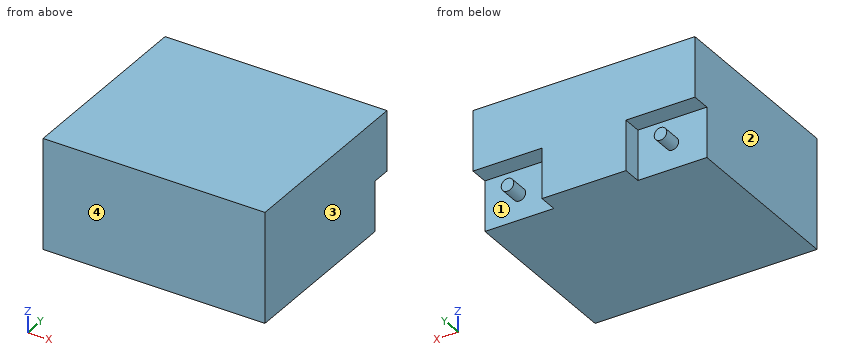
from build123d import *

# Parameters (mm, degrees)
F0_W     = 177
F0_H     = 154
F1_DEPTH = 88
F2_W     = 55
F2_H     = 40
F2_R     = 5
F3_DEPTH = 15


with BuildPart() as f1:
    # F0 (on Top) → F1 (new body)
    with BuildSketch(Plane.XY):
        with Locations((88.5, 77)):
            Rectangle(F0_W, F0_H)
    extrude(amount=F1_DEPTH)

    # F2 (on face) → F3 (cut)
    with BuildSketch(Plane(origin=(0, 154, 0), x_dir=(-1, 0, 0), z_dir=(0, 1, 0))):
        with Locations((-149.5, 20)):
            Rectangle(F2_W, F2_H)
        with Locations((-149.5, 20)):
            Circle(F2_R, mode=Mode.SUBTRACT)
        with Locations((-27.5, 20)):
            Rectangle(F2_W, F2_H)
        with Locations((-27.5, 20)):
            Circle(F2_R, mode=Mode.SUBTRACT)
    extrude(amount=-F3_DEPTH, mode=Mode.SUBTRACT)


solid = f1.part
The listing builds one solid part. Answer for the finished solid, in the listing's coordinates (mm). Face numbers are marked on the shaded views. Give positions to 0.01 mm unless a question says otherwise; leave off trailing zeros. Loops run counter-clockwise (first coordinate to the right, second up) from the corner with the lowest first, then second, coordinate; pieces in that order, holes last. Notation, with made-up numbers: (50, -18.5) - (96, -18.5) arc R33 cw to (96, 12.5) - close; hole circle Ø5 at (2.25, 24.5). An arc over 180 degrees is marked (long way). Use one line per item in the form item = value.
1. Find the intervals of material crossed by line 1 along Y through (x, z) = (48, 30); line 2 along X through (y, z) = (144.5, 12.5), in increasing order. Write a range as [from, to].
Calculated:
line_1 = [0, 139]
line_2 = [55, 122]
2. The mould has two halves that part along X. Classify the marked faces 1, 2, 3 and 4: pulls with the +X half, pulls with the -X half, needs draft (parallel to the pull), parting line crosses it, or undercut.
Calculated:
face_1 = undercut
face_2 = pulls with the -X half
face_3 = pulls with the +X half
face_4 = needs draft
3. Section B-B on x = 149.5 is taken. Give the vertices of the cut face in (y, z), then the cut area to 3 significant figures.
Calculated:
outline = (0, 0) - (139, 0) - (139, 15) - (154, 15) - (154, 25) - (139, 25) - (139, 40) - (154, 40) - (154, 88) - (0, 88) - close
area = 13,100 mm^2
4. Given pin 1 Ø12 at (x, y) = (28.5, 146.5) entering from -Z; pin 2 Ø12 at (x, z) = (156.5, 31.5) entering from +Y; pin 3 Ø7.5 at (y, z) = (144, 24.5) entering from +X, each flat-ended and moving along its own axis, determine where each tip first touches the part or whether it passes through.
Calculated:
pin_1 = 15
pin_2 = 139
pin_3 = 154.44
5. Section A-A on z = 20 is taken. Give the vertices of the cut face in (x, y), then the cut area to 3 significant figures.
Calculated:
outline = (0, 0) - (177, 0) - (177, 139) - (154.5, 139) - (154.5, 154) - (144.5, 154) - (144.5, 139) - (122, 139) - (122, 154) - (55, 154) - (55, 139) - (32.5, 139) - (32.5, 154) - (22.5, 154) - (22.5, 139) - (0, 139) - close
area = 25,900 mm^2
6. Section C-C on x = 124.5 is taken. Give the vertices of the cut face in (y, z), then the cut area to 3 significant figures.
Calculated:
outline = (0, 0) - (139, 0) - (139, 40) - (154, 40) - (154, 88) - (0, 88) - close
area = 13,000 mm^2
